The model under review builds one solid part; all positions refer to its coordinate system, in mm. A direction names the side the tool comes from. Round coordinates to 2 decimals unless told otherwise and drop trailing zeros. Write each loop counter-clockwise with the first axis right and the second up, starting at its lowest first coordinate (ties: lowest second). Pieces come first, ordered by that corner, then holes. Notation, with made-up numbers: (70, 7) - (122, 7) arc R11 ccw to (122, 25) - close; hole circle Ø11 at (-29.75, 33.25). An arc over 180 degrees is marked (long way). Return JSON: item names as keys, results as strings.
from build123d import *

# Parameters (mm, degrees)
F0_W     = 856.515822627
F0_H     = 50.8
F3_DEPTH = 25.4
F4_DEPTH = 0.508


with BuildPart() as f1:
    # F0 (on Right) → F1 (revolve)
    with BuildSketch(Plane.YZ):
        Rectangle(F0_W, F0_H)
    revolve(axis=Axis((0, 0, 25.4), (0, -1, 0)))

    # F2 (on face) → F3 (join)
    with BuildSketch(Plane.XZ.offset(428.2579113135)):
        with BuildLine():
            Line((-4.7912972498, 75.9735451661), (-4.7912972498, -25.1735451661))
            ThreePointArc((-4.7912972498, -25.1735451661), (-2.3983229103, -25.3433547099), (0, -25.4))
            ThreePointArc((0, -25.4), (2.3983229103, -25.3433547099), (4.7912972498, -25.1735451661))
            Line((4.7912972498, -25.1735451661), (4.7912972498, 75.9735451661))
            Line((4.7912972498, 75.9735451661), (0, 76.2))
            Line((0, 76.2), (-4.7912972498, 75.9735451661))
        make_face()
    extrude(amount=F3_DEPTH)

    # F2 (on face) → F4 (join)
    with BuildSketch(Plane.XZ.offset(428.2579113135)):
        with BuildLine():
            Line((-4.7912972498, 75.9735451661), (-4.7912972498, -25.1735451661))
            ThreePointArc((-4.7912972498, -25.1735451661), (-2.3983229103, -25.3433547099), (0, -25.4))
            ThreePointArc((0, -25.4), (2.3983229103, -25.3433547099), (4.7912972498, -25.1735451661))
            Line((4.7912972498, -25.1735451661), (4.7912972498, 75.9735451661))
            Line((4.7912972498, 75.9735451661), (0, 76.2))
            Line((0, 76.2), (-4.7912972498, 75.9735451661))
        make_face()
    extrude(amount=-F4_DEPTH)


solid = f1.part
(1) Add section D-D (x = 33). Write out the cut boundary in (y, z), plus the area to 3 significant figures.
Filled in:
{"outline": "(-428.26, -13.22) - (428.26, -13.22) - (428.26, 64.02) - (-428.26, 64.02) - close", "area": "66,200 mm2"}
(2) Wall thickness on line 1 (Y direction, x = -6, z = 40.5); line 2 (Z direction, x = 44, y = 359); line 3 (Z direction, x = 5, y = -380.5): over which ranges is each line inside the solid? List them lowest first.
Filled in:
{"line 1": "y = -428.26 to 428.26", "line 2": "z = 0.01 to 50.79", "line 3": "z = -25.15 to 75.95"}
(3) For faces 1 (the flat face through (4.791, -441, 25)), 2 (the flat face through (1, 428.258, 26)), 3 (the flat face through (-22, -428.258, 26)), list the 3-axis set-ups (+Z, -Z, +X, -X, +Y, -Y) from which the entire face can be reached by the end or side of a thin tool; tool diameter is ignored.
Filled in:
{"face 1": "+Z, -Z, +X, -Y", "face 2": "+Z, -Z, +X, -X, +Y", "face 3": "+Z, -Z, -X, -Y"}
(4) Add section B-B (y = -273). Write out the cut boundary in (x, z), plus the area to 3 significant figures.
Filled in:
{"outline": "circle Ø101.6 at (0, 25.4)", "area": "8,110 mm2"}
(5) Add section C-C (z = 58.5). Write out the cut boundary in (x, y).
Filled in:
{"outline": "(-38.54, -428.26) - (-4.79, -428.26) - (-4.79, -453.66) - (4.79, -453.66) - (4.79, -428.26) - (38.54, -428.26) - (38.54, 428.26) - (-38.54, 428.26) - close"}
(6) Clearance check with flat-ended pins moving along their axes: pin 1 Ø5 at (x, z) = (-39.5, 27) entering from -Y; pin 2 Ø7.5 at (y, z) = (-445, 12) entering from +X; pin 3 Ø1.5 at (y, z) = (275.5, 4) entering from +X. State where each tip first meets the part, or that it passes through.
Filled in:
{"pin 1": "stops at y = -428.26", "pin 2": "stops at x = 4.79", "pin 3": "stops at x = 46.41"}
(7) Add section A-A (z = 25.4). Write out the cut boundary in (x, y).
Filled in:
{"outline": "(-50.8, -428.26) - (-4.79, -428.26) - (-4.79, -453.66) - (4.79, -453.66) - (4.79, -428.26) - (50.8, -428.26) - (50.8, 428.26) - (-50.8, 428.26) - close"}
